Could you check a few things on this drawing? It's one solid part, dimensions in mm from its lowest x, y, z. A direction names the side the tool comes from. Give positions to 0.01 mm unless a question says otherwise; leave off trailing zeros. Loops run counter-clockwise (first coordinate to the right, second up) from the corner with the lowest first, then second, coordinate; pieces in that order, holes last. Notation, with made-up numbers: (62, 14.25) - (97, 14.25) arc R16 ccw to (97, 41.25) - close; hole circle Ø1 at (-10, -6.5). An arc over 180 degrees is marked (long way). Answer as a JSON object with one key per item and string values.
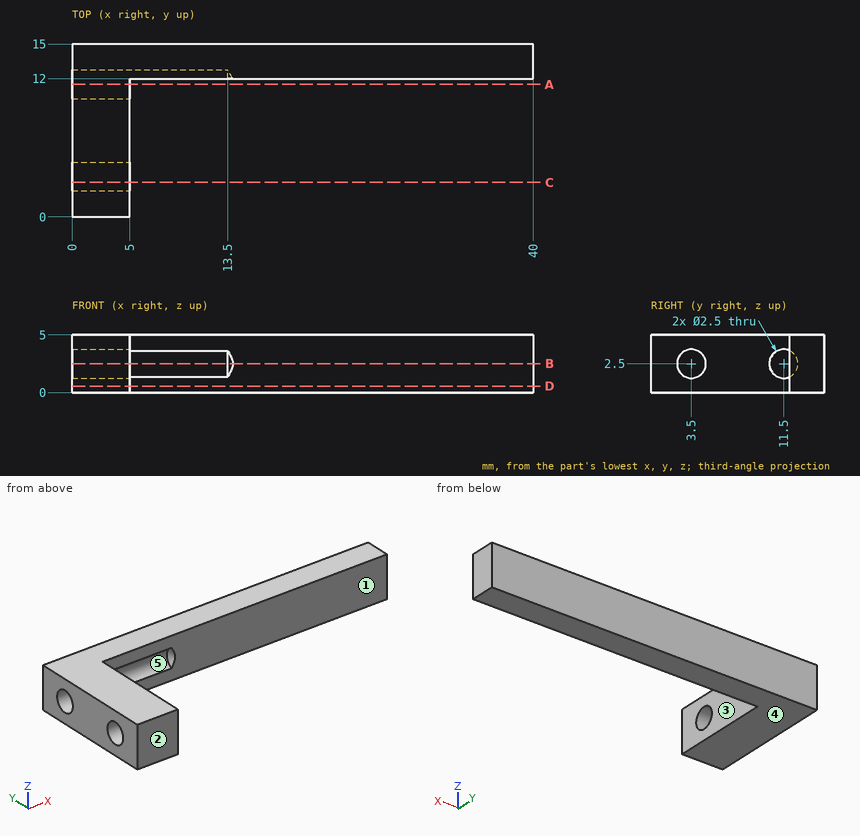
1) If we mould it in two halves opening along Z, with no side actions, what happens to the marked faces 3, 4 and 5? For each: released by +Z, released by -Z, zero draft, split by the parting line, or undercut.
Check sheet entries:
{"face 3": "zero draft", "face 4": "released by -Z", "face 5": "undercut"}
2) I need wall thicknesses on L1, parallel to Y at x = 1.75, z = 2.5; L2, parallel to Z at x = 3.5, y = 11.5; L3, parallel to X at y = 3.25, z = 4.25. Which ranges of each line are inside material? Lowest first, please.
Check sheet entries:
{"L1": "0 to 2.25, 4.75 to 10.25, 12.75 to 15", "L2": "0 to 1.25, 3.75 to 5", "L3": "0 to 5"}
3) Which directions (+Z, -Z, +X, -X, +Y, -Y) give clear straight access to the entire face, cutting with the end or side of a thin tool? Please do the marked faces 1 and 2.
Check sheet entries:
{"face 1": "+Z, -Z, +X, -Y", "face 2": "+Z, -Z, +X, -X, -Y"}
4) Imagine slicing it at D-D on z = 0.55. Write out the boundary of the cut face in (x, y).
Check sheet entries:
{"outline": "(0, 0) - (5, 0) - (5, 12) - (40, 12) - (40, 15) - (0, 15) - close"}
5) Imagine slicing it at B-B on z = 2.5. Write out the boundary of the cut face in (x, y), and give its area (3 significant figures).
Check sheet entries:
{"outline": "(0, 0) - (5, 0) - (5, 2.25) - (0, 2.25) - close; (0, 4.75) - (5, 4.75) - (5, 10.25) - (0, 10.25) - close; (0, 12.75) - (13.5, 12.75) - (13.95, 12) - (40, 12) - (40, 15) - (0, 15) - close", "area": "148 mm2"}
6) Imagine slicing it at A-A on y = 11.5. Write out the boundary of the cut face in (x, z).
Check sheet entries:
{"outline": "(0, 0) - (5, 0) - (5, 1.25) - (0, 1.25) - close; (0, 3.75) - (5, 3.75) - (5, 5) - (0, 5) - close"}
7) I'm going to push flat-ended pins straight in: P1, Ø1, axis at x = 23, y = 13, coming from the -Z side; P2, Ø2.5, axis at x = 25.5, z = 1.5, coming from the -Y side; P3, Ø1.5, axis at y = 11.5, z = 2.5, coming from the -X side. Where does each tip first touch, or does it pass through?
Check sheet entries:
{"P1": "z = 0", "P2": "y = 12", "P3": "x = 13.8"}
8) Imagine slicing it at C-C on y = 3. Write out the boundary of the cut face in (x, z), and give its area (3 significant figures).
Check sheet entries:
{"outline": "(0, 0) - (5, 0) - (5, 1.35) - (0, 1.35) - close; (0, 3.65) - (5, 3.65) - (5, 5) - (0, 5) - close", "area": "13.5 mm2"}
